Can you work these out from the model? Positions are in its coordinate system, mm. A direction names the side the tool comes from. Coordinates: 2 decimals unless noted, no trailing zeros. Loops run counter-clockwise (first coordinate to the right, second up) from the corner with the lowest first, then second, coordinate; pieces in that order, holes last. Notation, with made-up numbers: (83.5, -25.75) - (135.5, -25.75) arc R23 ccw to (135.5, 4.25) - close; hole circle Ø6 at (27.5, 52.25). An arc over 180 degrees is marked (long way). Put each result on its own line as item: value. Start each with the question number.
from build123d import *

# Parameters (mm, degrees)
SKETCH1_W           = 19
SKETCH1_H           = 22
BOSS_EXTRUDE1_DEPTH = 37
FILLET1_R           = 3.5
BOSS_EXTRUDE2_DEPTH = 19.5
BOSS_EXTRUDE3_DEPTH = 25


with BuildPart() as part:
    # Sketch1 → Boss-Extrude1 (new body)
    with BuildSketch(Plane(origin=(0, 0, 0), x_dir=(0, 1, 0), z_dir=(0, 0, 1))):
        with Locations((9.5, 11)):
            Rectangle(SKETCH1_W, SKETCH1_H)
    extrude(amount=BOSS_EXTRUDE1_DEPTH)

    # Fillet1
    fillet1_edges = [part.edges().sort_by_distance(p)[0] for p in [
        (-22, 9.5, 0),
        (0, 9.5, 0),
    ]]
    fillet(fillet1_edges, radius=FILLET1_R)

    # Sketch2 → Boss-Extrude2 (add, symmetric)
    with BuildSketch(Plane(origin=(0, 9.5, 0), x_dir=(1, 0, 0), z_dir=(0, 1, 0))):
        with BuildLine():
            Line((-12.75, -9.214642893), (-12.75, -11))
            Line((-12.75, -11), (-12.75, -12.785357107))
            ThreePointArc((-12.75, -12.785357107), (-11, -13.5), (-9.25, -12.785357107))
            Line((-9.25, -12.785357107), (-9.25, -11))
            Line((-9.25, -11), (-9.25, -9.214642893))
            ThreePointArc((-9.25, -9.214642893), (-11, -8.5), (-12.75, -9.214642893))
        make_face()
    extrude(amount=BOSS_EXTRUDE2_DEPTH, both=True)

    # Sketch4 → Boss-Extrude3 (add)
    with BuildSketch(Plane.XY.offset(37)):
        with BuildLine():
            Line((-7.877501001, 19), (-11, 19))
            Line((-11, 19), (-11, 0))
            Line((-11, 0), (-7.877501001, 0))
            ThreePointArc((-7.877501001, 0), (-2.899845989, 3.635913967), (-1, 9.5))
            ThreePointArc((-1, 9.5), (-2.899845989, 15.364086033), (-7.877501001, 19))
        make_face()
        with BuildLine():
            Line((-11, 0), (-11, 19))
            Line((-11, 19), (-14.122498999, 19))
            ThreePointArc((-14.122498999, 19), (-21, 9.5), (-14.122498999, 0))
            Line((-14.122498999, 0), (-11, 0))
        make_face()
    extrude(amount=BOSS_EXTRUDE3_DEPTH)


solid = part.part
Q1. I want a section at B-B on x = -15.75. List the corners of the cut face in (y, z) for me.
Q2. I want a section at D-D on x = -10.75. List the corners of the cut face in (y, z) for me, and give its area (3 significant figures).
Q3. Please list where these lines run through material, in increasing order: line 1 along Y through (x, z) = (-19.75, 17.5); line 2 along X through (y, z) = (3, 43); line 3 along Z through (x, y) = (-19.75, 7.5). Write a range as [from, to].
Q4. Will these pins go through, and if not, where does the flat tip stop? pin 1 (1.8 mm diameter, centred on y = -5.5, z = 11.5, fed in from -X); pin 2 (3 mm diameter, centred on y = 21.5, z = 10.5, fed in from +X); pin 3 (1 mm diameter, centred on x = -18.5, z = 38.5, fed in from -Y).
Q5. I want a section at C-C on z = 46.5. List the corners of the cut face in (x, y) for me, and give its area (3 significant figures).
Q6. I want a section at A-A on y = 15.5. List the corners of the cut face in (x, z) for me, and give its area (3 significant figures).
Q7. On a 3-axis mill with a long thin cutter (end or side, diameter ignored), from which of +Z, -Z, +X, -X, +Y, -Y can I reach the whole of each face in a straight line? I mean faces 1 (the flat face through (-12.75, -5, 11)), 2 (the flat face through (-0.2, 9.5, 37)), 3 (the cylindrical face through (-11, 24.1, 8.5)), 4 (the cylindrical face through (-11, -4.9, 8.5)), 5 (the flat face through (-12.75, 24, 11)). Say none if no direction works.
Calculated:
1. outline: (0, 0) - (19, 0) - (19, 37) - (18.3, 37) - (18.3, 62) - (0.7, 62) - (0.7, 37) - (0, 37) - close
2. outline: (-10, 8.51) - (0, 8.51) - (0, 0) - (19, 0) - (19, 8.51) - (29, 8.51) - (29, 13.49) - (19, 13.49) - (19, 62) - (0, 62) - (0, 13.49) - (-10, 13.49) - close
2. area: 1,280 mm2
3. line 1: [0, 19]
3. line 2: [-18.6, -3.4]
3. line 3: [0.23, 62]
4. pin 1: x = -12.75
4. pin 2: x = -9.25
4. pin 3: y = 2.36
5. outline: (-14.12, 0) - (-7.88, 0) arc R10 ccw to (-7.88, 19) - (-14.12, 19) arc R10 ccw to start
5. area: 310 mm2
6. outline: (-22, 3.5) arc R3.5 ccw to (-18.5, 0) - (-3.5, 0) arc R3.5 ccw to (0, 3.5) - (0, 37) - (-3, 37) - (-3, 62) - (-19, 62) - (-19, 37) - (-22, 37) - close
6. area: 1,210 mm2
7. face 1: +Z, -Z, -X, -Y
7. face 2: +Z, +X
7. face 3: -Z, +Y
7. face 4: -Z, -Y
7. face 5: +Z, -Z, -X, +Y
